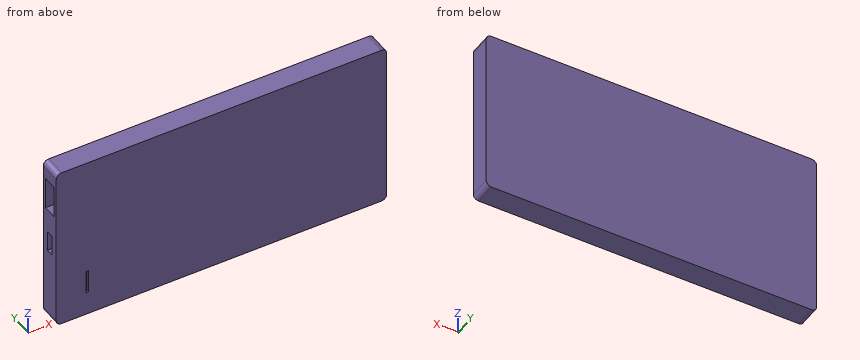
```python
from build123d import *

# Parameters (mm, degrees)
SKETCH1_W           = 124.65
SKETCH1_H           = 63.65
BOSS_EXTRUDE1_DEPTH = 8.2
SKETCH2_W           = 7.72
SKETCH2_H           = 2.7
SKETCH2_W_2         = 12.3
SKETCH2_H_2         = 5.3
CUT_EXTRUDE1_DEPTH  = 12
SKETCH3_W           = 1
SKETCH3_H           = 9
CUT_EXTRUDE2_DEPTH  = 1
FILLET1_R           = 2


with BuildPart() as part:
    # Sketch1 → Boss-Extrude1 (new body)
    with BuildSketch(Plane(origin=(0, 0, 0), x_dir=(1, 0, 0), z_dir=(0, 1, 0))):
        with Locations((4.430687204, 1.109774882)):
            Rectangle(SKETCH1_W, SKETCH1_H)
    extrude(amount=BOSS_EXTRUDE1_DEPTH)

    # Sketch2 → Cut-Extrude1 (cut)
    with BuildSketch(Plane.ZY.offset(57.894312796)):
        with Locations((-1.109774882, 4.1)):
            Rectangle(SKETCH2_W, SKETCH2_H)
        with Locations((18.220036332, 4.1)):
            Rectangle(SKETCH2_W_2, SKETCH2_H_2)
    extrude(amount=-CUT_EXTRUDE1_DEPTH, mode=Mode.SUBTRACT)

    # Sketch3 → Cut-Extrude2 (cut)
    with BuildSketch(Plane.XZ):
        with Locations((-46.194312796, -19.434774882)):
            Rectangle(SKETCH3_W, SKETCH3_H)
    extrude(amount=-CUT_EXTRUDE2_DEPTH, mode=Mode.SUBTRACT)

    # Fillet1
    fillet1_edges = [part.edges().sort_by_distance(p)[0] for p in [
        (-57.894312796, 4.1, -32.934774882),
        (66.755687204, 4.1, -32.934774882),
        (66.755687204, 4.1, 30.715225118),
        (-57.894312796, 4.1, 30.715225118),
    ]]
    fillet(fillet1_edges, radius=FILLET1_R)


solid = part.part
```
CAD build for the part. Positions are in the model's coordinates, mm. Round coordinates to 2 decimals unless told otherwise and drop trailing zeros. Order: outer loops, then holes, each group sorted by start corner. A loop starts at its lowest first (then second) coordinate and runs counter-clockwise, first axis right, second up. Notation, with made-up numbers: (-32.75, 42.25) - (-0.75, 42.25) arc R28 cw to (-0.75, 79.25) - close; hole circle Ø4 at (60.25, -21). An arc over 180 degrees is marked (long way). Answer as CSV lines item,"result". Start each with the question number.
1. Pin check, flat tip, straight feed: pin 1 (2.5 mm diameter, centred on y = 3, z = 20, fed in from -X). Stop position of the tip, or through.
2. Saw through at B-B, the plane z = 21.5. Write the cut outline in (x, y), and give its area (3 significant figures).
3. Saw through at C-C, the plane z = 1. Write the cut outline in (x, y), and give its area (3 significant figures).
4. Saw through at A-A, the plane y = 4. Write the cut outline in (x, z), and give its area (3 significant figures).
5. Drill centre line: L1, parallel to X at y = 2.5, z = 14.5. Where is it in solid material? Low to high. Write a range as [from, to].
Model answer:
1,pin 1,"stops at x = -45.89"
2,outline,"(-57.89, 0) - (66.76, 0) - (66.76, 8.2) - (-57.89, 8.2) - (-57.89, 6.75) - (-45.89, 6.75) - (-45.89, 1.45) - (-57.89, 1.45) - close"
2,area,"959 mm²"
3,outline,"(-57.89, 0) - (66.76, 0) - (66.76, 8.2) - (-57.89, 8.2) - (-57.89, 5.45) - (-45.89, 5.45) - (-45.89, 2.75) - (-57.89, 2.75) - close"
3,area,"990 mm²"
4,outline,"(-57.89, -30.93) arc R2 ccw to (-55.89, -32.93) - (64.76, -32.93) arc R2 ccw to (66.76, -30.93) - (66.76, 28.72) arc R2 ccw to (64.76, 30.72) - (-55.89, 30.72) arc R2 ccw to (-57.89, 28.72) - (-57.89, 24.37) - (-45.89, 24.37) - (-45.89, 12.07) - (-57.89, 12.07) - (-57.89, 2.75) - (-45.89, 2.75) - (-45.89, -4.97) - (-57.89, -4.97) - close"
4,area,"7,690 mm²"
5,L1,"x = [-45.89, 66.76]"
